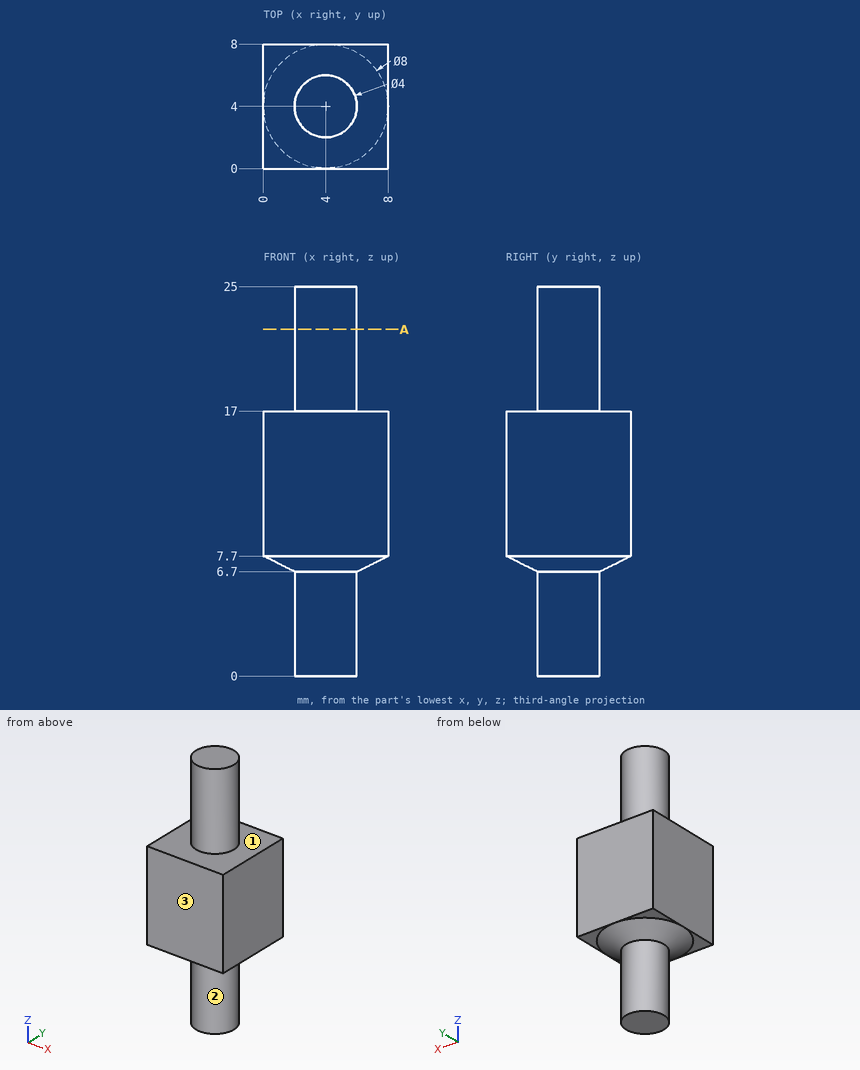
Could you check a few things on this drawing? It's one solid part, dimensions in mm from its lowest x, y, z. A direction names the side the tool comes from. Give positions to 0.01 mm unless a question says otherwise; leave off trailing zeros. Write each loop counter-clockwise with the first axis right and the second up, starting at its lowest first coordinate (ties: lowest second). Pieces come first, ordered by that corner, then holes. Notation, with made-up numbers: (86, -10) - (93, -10) arc R8 ccw to (93, 2) - close; hole circle Ø5 at (64.25, -11.5). An arc over 180 degrees is marked (long way). Use CSV: the item, a comma, the result in double quotes. Start each with the question number.
Item 1: For the marked faces 1, 2 and 3, which set-ups out of +Z, -Z, +X, -X, +Y, -Y let a thin tool reach every point of the face, with its end or its side?
Item 2: I'm going to push flat-ended pins straight in: pin 1 (1.5 mm diameter, centred on x = 3.5, z = 3.5, fed in from -Y); pin 2 (1.2 mm diameter, centred on x = 1, y = 6, fed in from -Z). Where does each tip first touch, or does it pass through?
Item 3: I want a section at A-A, the plane z = 22.25. Please give me the cut outline in (x, y).
Item 4: If I drill on line 1 along Y through (x, z) = (4, 22.75); line 2 along Z through (x, y) = (0.75, 7); line 3 along Y through (x, z) = (5.5, 20), over which ranges is the centre line in solid material (lowest first)?
Findings:
1,face 1,"+Z"
1,face 2,"-Z"
1,face 3,"+Z, -Z, +X, -X, -Y"
2,pin 1,"stops at y = 2"
2,pin 2,"stops at z = 7.2"
3,outline,"circle Ø4 at (4, 4)"
4,line 1,"y = 2 to 6"
4,line 2,"z = 7.7 to 17"
4,line 3,"y = 2.68 to 5.32"
